```python
from build123d import *

# Parameters (mm, degrees)
SKETCH1_R           = 9.144
BOSS_EXTRUDE1_DEPTH = 17.018
SKETCH2_W           = 14.986
SKETCH2_H           = 16.764
BOSS_EXTRUDE2_DEPTH = 20.32
SKETCH3_R           = 6.35
BOSS_EXTRUDE3_DEPTH = 20.828
SKETCH5_R           = 4.953
CUT_EXTRUDE1_DEPTH  = 25.4
SKETCH6_R           = 6.985
CUT_EXTRUDE2_DEPTH  = 35.56
FILLET3_R           = 2.54


with BuildPart() as part:
    # Sketch1 → Boss-Extrude1 (new body)
    with BuildSketch(Plane(origin=(0, 0, 0), x_dir=(1, 0, 0), z_dir=(0, 1, 0))):
        with Locations(Location((-13.844609685, 2.253750912, 0), (0, 0, 270))):
            Circle(SKETCH1_R)
    extrude(amount=BOSS_EXTRUDE1_DEPTH)

    # Sketch2 → Boss-Extrude2 (add)
    with BuildSketch(Plane(origin=(0, 17.018, 0), x_dir=(1, 0, 0), z_dir=(0, 1, 0))):
        with Locations((-13.844609685, 2.253750912)):
            Rectangle(SKETCH2_W, SKETCH2_H)
    extrude(amount=BOSS_EXTRUDE2_DEPTH)

    # Sketch3 → Boss-Extrude3 (add)
    with BuildSketch(Plane.XY.offset(6.128249088)):
        with Locations(Location((-13.844609685, 29.845, 0), (0, 0, 180))):
            Circle(SKETCH3_R)
    extrude(amount=BOSS_EXTRUDE3_DEPTH)

    # Sketch5 → Cut-Extrude1 (cut)
    with BuildSketch(Plane.XY.offset(26.956249088)):
        with Locations((-13.844609685, 29.845)):
            Circle(SKETCH5_R)
    extrude(amount=-CUT_EXTRUDE1_DEPTH, mode=Mode.SUBTRACT)

    # Sketch6 → Cut-Extrude2 (cut)
    with BuildSketch(Plane.XZ):
        with Locations(Location((-13.947920493, -2.516662253, 0), (0, 0, 270))):
            Circle(SKETCH6_R)
    extrude(amount=-CUT_EXTRUDE2_DEPTH, mode=Mode.SUBTRACT)

    # Fillet3
    # the kernel refuses this fillet: 2.54 mm, written as the material it takes off along each edge
    with BuildSketch(Plane(origin=(-13.844609685, 17.018, -2.253750912), x_dir=(-0.2627084277127984, 0, -0.9648752675909303), z_dir=(0.9648752675909303, 0, -0.2627084277127984))) as fillet3_piece_1_section:
        with BuildLine():
            CenterArc((9.144 - FILLET3_R, -FILLET3_R), FILLET3_R, 0, 90)
            Line((9.144 - FILLET3_R, 0), (9.144, 0))
            Line((9.144, 0), (9.144, -FILLET3_R))
        make_face()
    fillet3_piece_1 = revolve(axis=Axis((-13.844609685, 17.018, -2.253750912), (0, 1, 0)), revolution_arc=149.538336895, mode=Mode.PRIVATE)
    fillet3_piece_1 = split(fillet3_piece_1, bisect_by=Plane(origin=(-16.671949394, 16.123690595, -10.635750912), z_dir=(0, 0, -1)), keep=Keep.TOP, mode=Mode.PRIVATE)
    add(fillet3_piece_1, mode=Mode.SUBTRACT)
    with BuildSketch(Plane(origin=(-13.844609685, 17.018, -2.253750912), x_dir=(-0.2627084277127984, 0, -0.9648752675909303), z_dir=(0.9648752675909303, 0, -0.2627084277127984))) as fillet3_piece_2_section:
        with BuildLine():
            CenterArc((9.144 - FILLET3_R, -FILLET3_R), FILLET3_R, 0, 90)
            Line((9.144 - FILLET3_R, 0), (9.144, 0))
            Line((9.144, 0), (9.144, -FILLET3_R))
        make_face()
    fillet3_piece_2 = revolve(axis=Axis((-13.844609685, 17.018, -2.253750912), (0, 1, 0)), revolution_arc=149.538336895, mode=Mode.PRIVATE)
    fillet3_piece_2 = split(fillet3_piece_2, bisect_by=Plane(origin=(-16.671949372, 16.123690833, 6.128249088), z_dir=(0, 0, 1)), keep=Keep.TOP, mode=Mode.PRIVATE)
    add(fillet3_piece_2, mode=Mode.SUBTRACT)
    with BuildSketch(Plane(origin=(-13.844609685, 17.018, -2.253750912), x_dir=(-0.2627084277127984, 0, -0.9648752675909303), z_dir=(0.9648752675909303, 0, -0.2627084277127984))) as fillet3_piece_3_section:
        with BuildLine():
            CenterArc((9.144 - FILLET3_R, -FILLET3_R), FILLET3_R, 0, 90)
            Line((9.144 - FILLET3_R, 0), (9.144, 0))
            Line((9.144, 0), (9.144, -FILLET3_R))
        make_face()
    fillet3_piece_3 = revolve(axis=Axis((-13.844609685, 17.018, -2.253750912), (0, 1, 0)), revolution_arc=149.538336895, mode=Mode.PRIVATE)
    fillet3_piece_3 = split(fillet3_piece_3, bisect_by=Plane(origin=(-21.337609685, 16.368354177, -2.253748905), z_dir=(-1, 0, 0)), keep=Keep.TOP, mode=Mode.PRIVATE)
    add(fillet3_piece_3, mode=Mode.SUBTRACT)
    with BuildSketch(Plane(origin=(-13.844609685, 17.018, -2.253750912), x_dir=(-0.8937341447307489, 0, 0.4485970112945439), z_dir=(-0.4485970112945439, 0, -0.8937341447307489))) as fillet3_piece_4_section:
        with BuildLine():
            CenterArc((9.144 - FILLET3_R, -FILLET3_R), FILLET3_R, 0, 90)
            Line((9.144 - FILLET3_R, 0), (9.144, 0))
            Line((9.144, 0), (9.144, -FILLET3_R))
        make_face()
    fillet3_piece_4 = revolve(axis=Axis((-13.844609685, 17.018, -2.253750912), (0, 1, 0)), revolution_arc=63.346294775, mode=Mode.PRIVATE)
    fillet3_piece_4 = split(fillet3_piece_4, bisect_by=Plane(origin=(-21.337609685, 16.206370087, 2.181832168), z_dir=(-1, 0, 0)), keep=Keep.TOP, mode=Mode.PRIVATE)
    add(fillet3_piece_4, mode=Mode.SUBTRACT)
    with BuildSketch(Plane(origin=(-13.844609685, 17.018, -2.253750912), x_dir=(-0.8937341447307489, 0, 0.4485970112945439), z_dir=(-0.4485970112945439, 0, -0.8937341447307489))) as fillet3_piece_5_section:
        with BuildLine():
            CenterArc((9.144 - FILLET3_R, -FILLET3_R), FILLET3_R, 0, 90)
            Line((9.144 - FILLET3_R, 0), (9.144, 0))
            Line((9.144, 0), (9.144, -FILLET3_R))
        make_face()
    fillet3_piece_5 = revolve(axis=Axis((-13.844609685, 17.018, -2.253750912), (0, 1, 0)), revolution_arc=63.346294775, mode=Mode.PRIVATE)
    fillet3_piece_5 = split(fillet3_piece_5, bisect_by=Plane(origin=(-15.321370262, 16.241743505, 6.128249088), z_dir=(0, 0, 1)), keep=Keep.TOP, mode=Mode.PRIVATE)
    add(fillet3_piece_5, mode=Mode.SUBTRACT)
    with BuildSketch(Plane(origin=(-13.844609685, 17.018, -2.253750912), x_dir=(0.8937598579171911, 0, -0.4485457795764468), z_dir=(0.4485457795764468, 0, 0.8937598579171911))) as fillet3_piece_6_section:
        with BuildLine():
            CenterArc((9.144 - FILLET3_R, -FILLET3_R), FILLET3_R, 0, 90)
            Line((9.144 - FILLET3_R, 0), (9.144, 0))
            Line((9.144, 0), (9.144, -FILLET3_R))
        make_face()
    fillet3_piece_6 = revolve(axis=Axis((-13.844609685, 17.018, -2.253750912), (0, 1, 0)), revolution_arc=126.699158212, mode=Mode.PRIVATE)
    fillet3_piece_6 = split(fillet3_piece_6, bisect_by=Plane(origin=(-6.351609685, 16.206428058, -6.689039599), z_dir=(1, 0, 0)), keep=Keep.TOP, mode=Mode.PRIVATE)
    add(fillet3_piece_6, mode=Mode.SUBTRACT)
    with BuildSketch(Plane(origin=(-13.844609685, 17.018, -2.253750912), x_dir=(0.8937598579171911, 0, -0.4485457795764468), z_dir=(0.4485457795764468, 0, 0.8937598579171911))) as fillet3_piece_7_section:
        with BuildLine():
            CenterArc((9.144 - FILLET3_R, -FILLET3_R), FILLET3_R, 0, 90)
            Line((9.144 - FILLET3_R, 0), (9.144, 0))
            Line((9.144, 0), (9.144, -FILLET3_R))
        make_face()
    fillet3_piece_7 = revolve(axis=Axis((-13.844609685, 17.018, -2.253750912), (0, 1, 0)), revolution_arc=126.699158212, mode=Mode.PRIVATE)
    fillet3_piece_7 = split(fillet3_piece_7, bisect_by=Plane(origin=(-21.337609685, 16.206428241, -6.68903958), z_dir=(-1, 0, 0)), keep=Keep.TOP, mode=Mode.PRIVATE)
    add(fillet3_piece_7, mode=Mode.SUBTRACT)
    with BuildSketch(Plane(origin=(-13.844609685, 17.018, -2.253750912), x_dir=(0.8937598579171911, 0, -0.4485457795764468), z_dir=(0.4485457795764468, 0, 0.8937598579171911))) as fillet3_piece_8_section:
        with BuildLine():
            CenterArc((9.144 - FILLET3_R, -FILLET3_R), FILLET3_R, 0, 90)
            Line((9.144 - FILLET3_R, 0), (9.144, 0))
            Line((9.144, 0), (9.144, -FILLET3_R))
        make_face()
    fillet3_piece_8 = revolve(axis=Axis((-13.844609685, 17.018, -2.253750912), (0, 1, 0)), revolution_arc=126.699158212, mode=Mode.PRIVATE)
    fillet3_piece_8 = split(fillet3_piece_8, bisect_by=Plane(origin=(-13.844610271, 16.241742489, -10.635750912), z_dir=(0, 0, -1)), keep=Keep.TOP, mode=Mode.PRIVATE)
    add(fillet3_piece_8, mode=Mode.SUBTRACT)
    with BuildSketch(Plane(origin=(-13.844609685, 17.018, -2.253750912), x_dir=(0.26270842771276587, 0, 0.9648752675909392), z_dir=(-0.9648752675909392, 0, 0.26270842771276587))) as fillet3_piece_9_section:
        with BuildLine():
            CenterArc((9.144 - FILLET3_R, -FILLET3_R), FILLET3_R, 0, 90)
            Line((9.144 - FILLET3_R, 0), (9.144, 0))
            Line((9.144, 0), (9.144, -FILLET3_R))
        make_face()
    fillet3_piece_9 = revolve(axis=Axis((-13.844609685, 17.018, -2.253750912), (0, 1, 0)), revolution_arc=149.538336895, mode=Mode.PRIVATE)
    fillet3_piece_9 = split(fillet3_piece_9, bisect_by=Plane(origin=(-11.017269976, 16.123690595, 6.128249088), z_dir=(0, 0, 1)), keep=Keep.TOP, mode=Mode.PRIVATE)
    add(fillet3_piece_9, mode=Mode.SUBTRACT)
    with BuildSketch(Plane(origin=(-13.844609685, 17.018, -2.253750912), x_dir=(0.26270842771276587, 0, 0.9648752675909392), z_dir=(-0.9648752675909392, 0, 0.26270842771276587))) as fillet3_piece_10_section:
        with BuildLine():
            CenterArc((9.144 - FILLET3_R, -FILLET3_R), FILLET3_R, 0, 90)
            Line((9.144 - FILLET3_R, 0), (9.144, 0))
            Line((9.144, 0), (9.144, -FILLET3_R))
        make_face()
    fillet3_piece_10 = revolve(axis=Axis((-13.844609685, 17.018, -2.253750912), (0, 1, 0)), revolution_arc=149.538336895, mode=Mode.PRIVATE)
    fillet3_piece_10 = split(fillet3_piece_10, bisect_by=Plane(origin=(-11.017269998, 16.123690833, -10.635750912), z_dir=(0, 0, -1)), keep=Keep.TOP, mode=Mode.PRIVATE)
    add(fillet3_piece_10, mode=Mode.SUBTRACT)
    with BuildSketch(Plane(origin=(-13.844609685, 17.018, -2.253750912), x_dir=(0.26270842771276587, 0, 0.9648752675909392), z_dir=(-0.9648752675909392, 0, 0.26270842771276587))) as fillet3_piece_11_section:
        with BuildLine():
            CenterArc((9.144 - FILLET3_R, -FILLET3_R), FILLET3_R, 0, 90)
            Line((9.144 - FILLET3_R, 0), (9.144, 0))
            Line((9.144, 0), (9.144, -FILLET3_R))
        make_face()
    fillet3_piece_11 = revolve(axis=Axis((-13.844609685, 17.018, -2.253750912), (0, 1, 0)), revolution_arc=149.538336895, mode=Mode.PRIVATE)
    fillet3_piece_11 = split(fillet3_piece_11, bisect_by=Plane(origin=(-6.351609685, 16.368354177, -2.253752919), z_dir=(1, 0, 0)), keep=Keep.TOP, mode=Mode.PRIVATE)
    add(fillet3_piece_11, mode=Mode.SUBTRACT)
    with BuildSketch(Plane(origin=(-13.844609685, 17.018, -2.253750912), x_dir=(0, 0, 1), z_dir=(-1, 0, 0))) as fillet3_piece_12_section:
        with BuildLine():
            CenterArc((9.144 - FILLET3_R, -FILLET3_R), FILLET3_R, 0, 90)
            Line((9.144 - FILLET3_R, 0), (9.144, 0))
            Line((9.144, 0), (9.144, -FILLET3_R))
        make_face()
    fillet3_piece_12 = revolve(axis=Axis((-13.844609685, 17.018, -2.253750912), (0, 1, 0)), revolution_arc=63.346294775, mode=Mode.PRIVATE)
    fillet3_piece_12 = split(fillet3_piece_12, bisect_by=Plane(origin=(-12.367849263, 16.241743644, 6.128249088), z_dir=(0, 0, 1)), keep=Keep.TOP, mode=Mode.PRIVATE)
    add(fillet3_piece_12, mode=Mode.SUBTRACT)
    with BuildSketch(Plane(origin=(-13.844609685, 17.018, -2.253750912), x_dir=(0, 0, 1), z_dir=(-1, 0, 0))) as fillet3_piece_13_section:
        with BuildLine():
            CenterArc((9.144 - FILLET3_R, -FILLET3_R), FILLET3_R, 0, 90)
            Line((9.144 - FILLET3_R, 0), (9.144, 0))
            Line((9.144, 0), (9.144, -FILLET3_R))
        make_face()
    fillet3_piece_13 = revolve(axis=Axis((-13.844609685, 17.018, -2.253750912), (0, 1, 0)), revolution_arc=63.346294775, mode=Mode.PRIVATE)
    fillet3_piece_13 = split(fillet3_piece_13, bisect_by=Plane(origin=(-6.351609685, 16.20637027, 2.181832149), z_dir=(1, 0, 0)), keep=Keep.TOP, mode=Mode.PRIVATE)
    add(fillet3_piece_13, mode=Mode.SUBTRACT)


solid = part.part
```
The model under review builds one solid part; all positions refer to its coordinate system, in mm. A direction names the side the tool comes from. Round coordinates to 2 decimals unless told otherwise and drop trailing zeros. Order: outer loops, then holes, each group sorted by start corner. A loop starts at its lowest first (then second) coordinate and runs counter-clockwise, first axis right, second up. Notation, with made-up numbers: M 41,76 L 67,76 A15 ccw 67,81 Z; hole C 31,-29 d2. An arc over 180 degrees is marked long. Use a Markdown table: item, result.
1) Tool access review of faces 4 (the face through (-7, 17.018, -10)), 5 (the face through (-13.02, 23.55, 16.4)), 6 (the face through (-20, 17.018, -10)): name each direction out of +Z, -Z, +X, -X, +Y, -Y from which nothing blocks a thin tool from reaching the whole face with its end or side.
Report:
| item | result |
|---|---|
| face 4 | -Z, +X, -Y |
| face 5 | +Z |
| face 6 | -Z, -X, -Y |
2) Consider section D-D (x = -18.25). Write out the cut boundary in (y, z).
Report:
| item | result |
|---|---|
| outline | M 0,-10.27 L 17.02,-10.27 L 17.02,-10.64 L 37.34,-10.64 L 37.34,6.13 L 34.42,6.13 L 34.42,26.96 L 32.11,26.96 L 32.11,2.99 L 35.56,2.99 L 35.56,-8.02 L 0,-8.02 Z; M 0,2.99 L 27.58,2.99 L 27.58,26.96 L 25.27,26.96 L 25.27,6.13 L 17.02,6.13 L 17.02,5.76 L 0,5.76 Z |
3) Draft analysis for pull direction Z (two halves, no side actions). For faces 1 (the face through (-16.62, 17.53, -8.97)), 2 (the face through (-7, 17.018, 5)), 3 (the face through (-13.44, 8.39, -11.39)), state which applies: released by +Z, released by -Z, zero draft, split by the parting line, or undercut.
Report:
| item | result |
|---|---|
| face 1 | undercut |
| face 2 | zero draft |
| face 3 | split by the parting line |
4) Consider section B-B (y = 34). Write out the cut boundary in (x, z) (3 decimals), then the cut area to 3 significant figures.
Report:
| item | result |
|---|---|
| outline | M -21.338,-10.636 L -6.352,-10.636 L -6.352,6.128 L -9.043,6.128 L -9.043,26.956 L -11.149,26.956 L -11.149,3.883 A6.985 cw long -16.541,3.969 L -16.541,26.956 L -18.647,26.956 L -18.647,6.128 L -21.338,6.128 Z |
| area | 176 mm^2 |
5) Wall thickness on line 1 along Z through (x, y) = (-19.5, 4.5); line 2 along Y through (x, z) = (-15, 10); line 3 along X through (y, z) = (10, -4.5): over which ranges is each line inside the solid? List them lowest first. Write a range as [from, to].
Report:
| item | result |
|---|---|
| line 1 | [-9.44, -6.76], [1.72, 4.93] |
| line 2 | [23.6, 25.03], [34.66, 36.09] |
| line 3 | [-22.71, -20.65], [-7.25, -4.98] |
6) Insertion check: pin 1 (5 mm diameter, centred on y = 30.5, z = 1.5, fed in from -X); pin 2 (10 mm diameter, centred on y = 21, z = -5, fed in from -X); pin 3 (2 mm diameter, centred on x = -18, y = 21.5, fed in from -Z). Each pin has a flat end and moves straight along its axis. Give the tip position at first contact, or say it passes through.
Report:
| item | result |
|---|---|
| pin 1 | x = -21.34 |
| pin 2 | x = -22.22 |
| pin 3 | z = -10.64 |
7) Consider section C-C (z = -8). Write out the cut boundary in (x, y), then the cut area to 3 significant figures.
Report:
| item | result |
|---|---|
| outline | M -21.34,17.02 L -20.96,17.02 L -20.96,0 L -18.27,0 L -18.27,35.56 L -9.62,35.56 L -9.62,0 L -6.73,0 L -6.73,17.02 L -6.35,17.02 L -6.35,37.34 L -21.34,37.34 Z |
| area | 239 mm^2 |
8) Consider section A-A (x = -9.5). Write out the cut boundary in (y, z).
Report:
| item | result |
|---|---|
| outline | M 0,-10.3 L 17.02,-10.3 L 17.02,-10.64 L 37.34,-10.64 L 37.34,6.13 L 34.48,6.13 L 34.48,26.96 L 32.22,26.96 L 32.22,2.87 L 35.56,2.87 L 35.56,-7.9 L 0,-7.9 Z; M 0,2.87 L 27.47,2.87 L 27.47,26.96 L 25.21,26.96 L 25.21,6.13 L 17.02,6.13 L 17.02,5.79 L 0,5.79 Z |
